Design review of the part built by this model. Coordinates are the model's own, in mm. A direction names the side the tool comes from. Give positions to 0.01 mm unless a question says otherwise; leave off trailing zeros. Loops run counter-clockwise (first coordinate to the right, second up) from the corner with the lowest first, then second, coordinate; pieces in that order, holes last. Notation, with made-up numbers: (25, 36) -> (43, 36) arc R21 ccw to (43, 74) -> close; hole circle Ø9 at (14, 36.5). An arc over 180 degrees is marked (long way). Use CSV: the item, a comma, the result in double quotes. Start each with the question number.
Item 1: For faces 1 (the face through (3, 5.08, -4)), 2 (the face through (0.213, 0.764, -14.516)), 3 (the face through (0, 12.7, 0)), list the 3-axis set-ups (+Z, -Z, +X, -X, +Y, -Y) from which the entire face can be reached by the end or side of a thin tool; tool diameter is ignored.
Item 2: We need section D-D (y = 11). State the section outline as (x, z) points.
Item 3: Wall thickness on line 1 along Z through (x, y) = (0, 8.5); line 2 along Z through (x, y) = (0, 4.5); line 3 along Y through (x, z) = (7.5, 10): over which ranges is each line inside the solid? List them lowest first. Write a range as from..to.
Item 4: We need section A-A (y = 3.5). State the section outline as (x, z) points, plus the area to 3 significant figures.
Item 5: We need section C-C (x = 0). State the section outline as (y, z) points, plus the area to 3 significant figures.
Item 6: We need section B-B (z = 0). State the section outline as (x, y) points, plus the area to 3 significant figures.
Item 7: The part is to be moulded in two halves that separate along Z. For faces 4 (the face through (15.24, 4, 0)), 5 (the face through (-0.33, 6.26, 2.52)), 6 (the face through (-0.83, 9.46, 3.72)), say which applies: +Z half, -Z half, draft (parallel to the pull), parting line (faces both ways), or undercut.
Item 8: Clearance check with flat-ended pins moving along their axes: pin 1 (6 mm diameter, centred on x = 0, z = 0, fed in from -Y); pin 2 (1 mm diameter, centred on x = -8, z = -5.5, fed in from +Y); pin 3 (1.5 mm diameter, centred on x = -1.5, z = 0.5, fed in from -Y). State where each tip first meets the part, or that it passes through.
from build123d import *

# Parameters (mm, degrees)
SKETCH1_W           = 30.48
SKETCH1_H           = 30.48
BOSS_EXTRUDE1_DEPTH = 5.08
SKETCH2_R           = 3.81
BOSS_EXTRUDE2_DEPTH = 8.89
FILLET1_R           = 2.54
SKETCH3_R           = 2.54
CUT_EXTRUDE1_DEPTH  = 12.7


with BuildPart() as part:
    # Sketch1 → Boss-Extrude1 (new body)
    with BuildSketch(Plane(origin=(0, 0, 0), x_dir=(1, 0, 0), z_dir=(0, 1, 0))):
        Rectangle(SKETCH1_W, SKETCH1_H)
    extrude(amount=BOSS_EXTRUDE1_DEPTH)

    # Sketch2 → Boss-Extrude2 (add)
    with BuildSketch(Plane(origin=(0, 5.08, 0), x_dir=(1, 0, 0), z_dir=(0, 1, 0))):
        Circle(SKETCH2_R)
    extrude(amount=BOSS_EXTRUDE2_DEPTH)

    # Fillet1
    fillet1_edges = [part.edges().sort_by_distance(p)[0] for p in [
        (0, 0, 15.24),
        (-15.24, 0, 0),
        (0, 0, -15.24),
        (15.24, 0, 0),
    ]]
    fillet(fillet1_edges, radius=FILLET1_R)

    # Sketch3 → Cut-Extrude1 (cut)
    with BuildSketch(Plane.XZ):
        Circle(SKETCH3_R)
    extrude(amount=-CUT_EXTRUDE1_DEPTH, mode=Mode.SUBTRACT)


solid = part.part
Results found:
1,face 1,"+Y"
1,face 2,"-Z, +X, -X, -Y"
1,face 3,"-Y"
2,outline,"circle Ø7.62 at (0, 0); hole circle Ø5.08 at (0, 0)"
3,line 1,"-3.81..-2.54, 2.54..3.81"
3,line 2,"-15.24..-2.54, 2.54..15.24"
3,line 3,"0..5.08"
4,outline,"(-15.24, -15.24) -> (15.24, -15.24) -> (15.24, 15.24) -> (-15.24, 15.24) -> close; hole circle Ø5.08 at (0, 0)"
4,area,"909 mm²"
5,outline,"(0, -12.7) arc R2.54 ccw to (2.54, -15.24) -> (5.08, -15.24) -> (5.08, -3.81) -> (13.97, -3.81) -> (13.97, 3.81) -> (5.08, 3.81) -> (5.08, 15.24) -> (2.54, 15.24) arc R2.54 ccw to (0, 12.7) -> (0, 2.54) -> (12.7, 2.54) -> (12.7, -2.54) -> (0, -2.54) -> close"
5,area,"155 mm²"
6,outline,"(-15.24, 2.54) arc R2.54 ccw to (-12.7, 0) -> (-2.54, 0) -> (-2.54, 12.7) -> (2.54, 12.7) -> (2.54, 0) -> (12.7, 0) arc R2.54 ccw to (15.24, 2.54) -> (15.24, 5.08) -> (3.81, 5.08) -> (3.81, 13.97) -> (-3.81, 13.97) -> (-3.81, 5.08) -> (-15.24, 5.08) -> close"
6,area,"155 mm²"
7,face 4,"draft"
7,face 5,"undercut"
7,face 6,"parting line"
8,pin 1,"y = 0"
8,pin 2,"y = 5.08"
8,pin 3,"y = 12.7"
